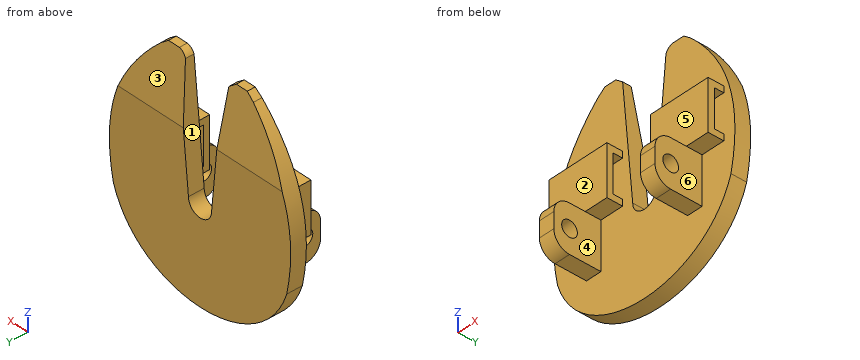
from build123d import *

# Parameters (mm, degrees)
BOSS_EXTRUDE1_DEPTH = 5
SKETCH2_W           = 20
SKETCH2_H           = 2
BOSS_EXTRUDE2_DEPTH = 3
SKETCH3_W           = 20
SKETCH3_H           = 16
BOSS_EXTRUDE3_DEPTH = 2
CUT_EXTRUDE1_DEPTH  = 62.362825506
SKETCH6_W           = 5
SKETCH6_H           = 15
BOSS_EXTRUDE4_DEPTH = 15
SKETCH7_R           = 2.5
CUT_EXTRUDE2_DEPTH  = 40
FILLET1_R           = 5
SKETCH8_W           = 2
SKETCH8_H           = 12
BOSS_EXTRUDE5_DEPTH = 3


with BuildPart() as part:
    # Sketch1 → Boss-Extrude1 (new body)
    with BuildSketch(Plane(origin=(0, 0, 0), x_dir=(1, 0, 0), z_dir=(0, 1, 0))):
        with BuildLine():
            Line((26, -9.914732545), (22.5, -47.146428929))
            Line((22.5, -47.146428929), (20.1411286, -49))
            Line((20.1411286, -49), (16.3588714, -49))
            Line((16.3588714, -49), (14, -47.146428929))
            add(Edge.make_bspline(
                [(0, 0), (-5.93850555, -28.119223668), (14, -47.146428929)],
                knots=[0, 0, 0, 1, 1, 1], degree=2))
            add(Edge.make_bspline(
                [(0, 0), (8.75, 26.780356607), (51.25, 26.780356607), (60, 0)],
                knots=[0, 0, 0, 0, 1, 1, 1, 1], degree=3))
            add(Edge.make_bspline(
                [(60, 0), (65.93850555, -28.119223668), (46, -47.146428929)],
                knots=[0, 0, 0, 1, 1, 1], degree=2))
            Line((46, -47.146428929), (43.6411286, -49))
            Line((43.6411286, -49), (39.8588714, -49))
            add(Edge.make_bspline(
                [(37.5, -47.146428929), (38.196873938, -48.687326951), (39.8588714, -49)],
                knots=[0, 0, 0, 1, 1, 1], degree=2))
            Line((37.5, -47.146428929), (34, -9.914732545))
            ThreePointArc((34, -9.914732545), (30, -5.914732545), (26, -9.914732545))
        make_face()
    extrude(amount=BOSS_EXTRUDE1_DEPTH)

    # Sketch2 → Boss-Extrude2 (add)
    with BuildSketch(Plane.XZ):
        with Locations((47.5, 11.914732545)):
            Rectangle(SKETCH2_W, SKETCH2_H)
        with Locations((47.5, 25.914732545)):
            Rectangle(SKETCH2_W, SKETCH2_H)
        with Locations((12.5, 11.914732545)):
            Rectangle(SKETCH2_W, SKETCH2_H)
        with Locations((12.5, 25.914732545)):
            Rectangle(SKETCH2_W, SKETCH2_H)
    extrude(amount=BOSS_EXTRUDE2_DEPTH)

    # Sketch3 → Boss-Extrude3 (add)
    with BuildSketch(Plane.XZ.offset(3)):
        with Locations((47.5, 18.914732545)):
            Rectangle(SKETCH3_W, SKETCH3_H)
        with Locations((12.5, 18.914732545)):
            Rectangle(SKETCH3_W, SKETCH3_H)
    extrude(amount=BOSS_EXTRUDE3_DEPTH)

    # Sketch5 → Cut-Extrude1 (cut, through all)
    with BuildSketch(Plane(origin=(0, 0, 0), x_dir=(0, 0, -1), z_dir=(1, 0, 0))):
        Polygon((-29, 5), (-49, 2.5), (-49, 5), align=None)
    extrude(amount=CUT_EXTRUDE1_DEPTH, mode=Mode.SUBTRACT)

    # Sketch6 → Boss-Extrude4 (add)
    with BuildSketch(Plane.XZ):
        with Locations((12.5, 3.414732545)):
            Rectangle(SKETCH6_W, SKETCH6_H)
    boss_extrude4 = extrude(amount=BOSS_EXTRUDE4_DEPTH)

    # Mirror1: Boss-Extrude4 across plane
    add(boss_extrude4.mirror(Plane(origin=(30, 0, 0), x_dir=(0, 0, 1), z_dir=(1, 0, 0))))

    # Sketch7 → Cut-Extrude2 (cut)
    with BuildSketch(Plane.ZY.offset(-10)):
        with Locations((3.414732545, -10)):
            Circle(SKETCH7_R)
    extrude(amount=-CUT_EXTRUDE2_DEPTH, mode=Mode.SUBTRACT)

    # Fillet1
    fillet1_edges = [part.edges().sort_by_distance(p)[0] for p in [
        (12.5, -15, 10.914732545),
        (12.5, -15, -4.085267455),
        (47.5, -15, 10.914732545),
        (47.5, -15, -4.085267455),
    ]]
    fillet(fillet1_edges, radius=FILLET1_R)

    # Sketch8 → Boss-Extrude5 (add)
    with BuildSketch(Plane.XZ):
        with Locations((3.5, 18.914732545)):
            Rectangle(SKETCH8_W, SKETCH8_H)
    extrude(amount=BOSS_EXTRUDE5_DEPTH)


solid = part.part
Check sheet for the modelled part. Datum: model origin and axes. Units: mm. Face numbers are marked on the shaded views. A direction names the side the tool comes from. Give positions to 0.01 mm unless a question says otherwise; leave off trailing zeros. Write each loop counter-clockwise with the first axis right and the second up, starting at its lowest first coordinate (ties: lowest second). Pieces come first, ordered by that corner, then holes. Notation, with made-up numbers: M 60.25,23 L 73.25,23 A23 cw 73.25,42 Z; hole C 47.25,75 d8. An arc over 180 degrees is marked long. Use one line per item in the form item = value.
(1) Draft check along X on the marked faces 4, 5 and 6. Enter one of: pulls with the +X half, pulls with the -X half, needs draft (parallel to the pull), parting line crosses it, or undercut.
Answer block:
face_4 = undercut
face_5 = needs draft
face_6 = pulls with the +X half
(2) Section check B-B on y = -11.25. Record the boundary of the cut face in (x, z).
Answer block:
outline = M 10,-3.93 L 15,-3.93 L 15,1.25 L 10,1.25 Z; M 10,5.58 L 15,5.58 L 15,10.76 L 10,10.76 Z; M 45,-3.93 L 50,-3.93 L 50,1.25 L 45,1.25 Z; M 45,5.58 L 50,5.58 L 50,10.76 L 45,10.76 Z
(3) Tool access check on the marked faces 1, 2 and 3. Record the directions out of +Z, -Z, +X, -X, +Y, -Y that give a thin tool (end or side, any length) a straight path to the whole face; none if there is none.
Answer block:
face_1 = +Z, +Y, -Y
face_2 = +Z, +X, -X, -Y
face_3 = +Z, +X, -X, +Y
(4) Section check A-A on y = -4. Record the boundary of the cut face in (x, z).
Answer block:
outline = M 2.5,10.91 L 10,10.91 L 10,-4.09 L 15,-4.09 L 15,10.91 L 22.5,10.91 L 22.5,26.91 L 2.5,26.91 Z; M 37.5,10.91 L 45,10.91 L 45,-4.09 L 50,-4.09 L 50,10.91 L 57.5,10.91 L 57.5,26.91 L 37.5,26.91 Z
(5) Material ranges on line 1 along Y through (x, z) = (32, -3.5); line 2 along X through (y, z) = (-14, -1); line 3 along X through (y, z) = (1, 20), recorded low to high.
Answer block:
line_1 = 0 to 5
line_2 = 10 to 15, 45 to 50
line_3 = -0.79 to 25.05, 34.95 to 60.79
(6) Depth check by flat-ended pin: P1, Ø8, axis at x = 8.5, z = 20, coming from the -Y side; P2, Ø12, axis at y = -8.5, z = 6.5, coming from the +X side; P3, Ø19, axis at x = 42.5, z = 16.5, coming from the -Y side. Enter the tip coordinate at first touch or a pass-through.
Answer block:
P1 = -5
P2 = 57.5
P3 = -14.79
